For this review, take the finished solid that the model builds, in its own axes (mm). Face numbers are marked on the shaded views. A direction names the side the tool comes from. Coordinates: 2 decimals unless noted, no trailing zeros. Loops run counter-clockwise (first coordinate to the right, second up) from the corner with the lowest first, then second, coordinate; pieces in that order, holes last. Notation, with made-up numbers: M -16,-1.5 L 37,-1.5 A12 ccw 37,16.5 Z; hole C 10.25,25.5 d5. An arc over 180 degrees is marked long. Use one line per item in the form item = value.
```python
from build123d import *

# Parameters (mm, degrees)
FILLET1_R = 15


with BuildPart() as part:
    # Sketch1 → Revolve1 (revolve)
    with BuildSketch(Plane.XY):
        Polygon((0, 72.092198582), (0, -13.907801418), (26.5, -13.907801418), (26.5, -12.907801418), (24, -9.907801418), (18, -9.907801418), (3, -9.907801418), (3, 5.092198582), (3, 72.092198582), align=None)
    revolve(axis=Axis((0, 72.092198582, 0), (0, -1, 0)))

    # Fillet1
    fillet1_edges = [part.edges().sort_by_distance(p)[0] for p in [
        (-3, -9.907801418, 0),
    ]]
    fillet(fillet1_edges, radius=FILLET1_R)


solid = part.part
```
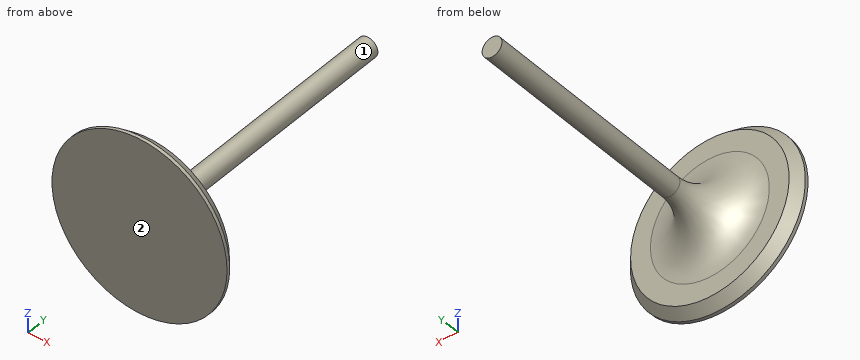
1. For pin 1 Ø3 at (x, z) = (-6.5, 11) entering from +Y; pin 2 Ø8 at (x, y) = (5.5, 45) entering from +Z, all flat-tipped, find the tip position at first contact; note any pin that passes through.
Computed values:
pin_1 = -8.32
pin_2 = 2.6
2. Tool access review of the marked faces 1 and 2: name each direction out of +Z, -Z, +X, -X, +Y, -Y from which nothing blocks a thin tool from reaching the whole face with its end or side.
Computed values:
face_1 = +Y
face_2 = +Z, -Z, +X, -X, -Y
3. Wall thickness on line 1 along Y through (x, z) = (10, 19); line 2 along Y through (x, z) = (9, -14); line 3 along Z through (x, y) = (-2, 60.5): over which ranges is each line inside the solid? List them lowest first. Write a range as from..to.
Computed values:
line_1 = -13.91..-9.91
line_2 = -13.91..-9.85
line_3 = -2.24..2.24
4. Consider section B-B on x = 0. Write out the cut boundary in (y, z), plus the area to 3 significant figures.
Computed values:
outline = M -13.91,-26.5 L -12.91,-26.5 L -9.91,-24 L -9.91,-18 A15 cw 5.09,-3 L 72.09,-3 L 72.09,3 L 5.09,3 A15 cw -9.91,18 L -9.91,24 L -12.91,26.5 L -13.91,26.5 Z
area = 793 mm2
5. Consider section C-C on y = 11. Write out the cut boundary in (x, z).
Computed values:
outline = C 0,0 d6
6. Consider section D-D on y = -7. Write out the cut boundary in (x, z).
Computed values:
outline = C 0,0 d18.25
7. Consider section A-A on z = 0. Write out the cut boundary in (x, y), plus the area to 3 significant figures.
Computed values:
outline = M -26.5,-13.91 L 26.5,-13.91 L 26.5,-12.91 L 24,-9.91 L 18,-9.91 A15 cw 3,5.09 L 3,72.09 L -3,72.09 L -3,5.09 A15 cw -18,-9.91 L -24,-9.91 L -26.5,-12.91 Z
area = 793 mm2
